For this review, take the finished solid that the model builds, in its own axes (mm). A direction names the side the tool comes from. Give positions to 0.01 mm unless a question says otherwise; leave off trailing zeros. Order: outer loops, then holes, each group sorted by start corner. A loop starts at its lowest first (then second) coordinate and runs counter-clockwise, first axis right, second up. Notation, with made-up numbers: (17, 85.5) - (76, 85.5) arc R30 cw to (76, 117.5) - close; hole circle Ø5 at (48.5, -25.5). An arc over 180 degrees is marked (long way). One line per item, written item: value.
```python
from build123d import *

# Parameters (mm, degrees)
CROQUIS1_R              = 5
SALIENTE_EXTRUIR1_DEPTH = 5
CROQUIS2_R              = 15
SALIENTE_EXTRUIR2_DEPTH = 5
CROQUIS3_R              = 1.5
CORTAR_EXTRUIR1_DEPTH   = 5
REDONDEO1_R             = 1
REDONDEO2_R             = 1


with BuildPart() as part:
    # Croquis1 → Saliente-Extruir1 (new, symmetric)
    with BuildSketch(Plane.XY):
        Circle(CROQUIS1_R)
        with BuildLine():
            Line((-2.236067977, -2), (2.236067977, -2))
            ThreePointArc((2.236067977, -2), (3, 0), (2.236067977, 2))
            Line((2.236067977, 2), (-2.236067977, 2))
            ThreePointArc((-2.236067977, 2), (-3, 0), (-2.236067977, -2))
        make_face(mode=Mode.SUBTRACT)
    extrude(amount=SALIENTE_EXTRUIR1_DEPTH, both=True)

    # Croquis2 → Saliente-Extruir2 (add)
    with BuildSketch(Plane(origin=(0, 0, -5), x_dir=(-1, 0, 0), z_dir=(0, 0, -1))):
        Circle(CROQUIS2_R)
    extrude(amount=SALIENTE_EXTRUIR2_DEPTH)

    # Croquis3 → Cortar-Extruir1 (cut)
    with BuildSketch(Plane.XY.offset(-5)):
        with Locations((-7.5, 7.5)):
            Circle(CROQUIS3_R)
        with Locations((7.5, 7.5)):
            Circle(CROQUIS3_R)
        with Locations((-7.5, -7.5)):
            Circle(CROQUIS3_R)
        with Locations((7.5, -7.5)):
            Circle(CROQUIS3_R)
    extrude(amount=-CORTAR_EXTRUIR1_DEPTH, mode=Mode.SUBTRACT)

    # Redondeo1
    redondeo1_edges = [part.edges().sort_by_distance(p)[0] for p in [
        (15, 0, -5),
    ]]
    fillet(redondeo1_edges, radius=REDONDEO1_R)

    # Redondeo2
    redondeo2_edges = [part.edges().sort_by_distance(p)[0] for p in [
        (-5, 0, 5),
    ]]
    fillet(redondeo2_edges, radius=REDONDEO2_R)


solid = part.part
```
(1) Take a section at B-B (y = 0). Write out the cut boundary in (x, z).
Answers below:
outline: (-15, -10) - (15, -10) - (15, -6) arc R1 ccw to (14, -5) - (5, -5) - (5, 4) arc R1 ccw to (4, 5) - (3, 5) - (3, -5) - (-3, -5) - (-3, 5) - (-4, 5) arc R1 ccw to (-5, 4) - (-5, -5) - (-14, -5) arc R1 ccw to (-15, -6) - close
(2) For P1, Ø5, axis at y = 3.5, z = -1, coming from the +X side; P2, Ø5, axis at x = 7.5, y = -7.5, coming from the +Z side; P3, Ø2, axis at x = 0.5, z = -1, coming from the +Y side, all flat-tipped, find the tip position at first contact; note any pin that passes through.
Answers below:
P1: stops at x = 4.9
P2: stops at z = -5
P3: stops at y = 5
(3) Wall thickness on line 1 (X direction, y = 6.5, z = -9.25); line 2 (Y direction, x = -7.5, z = -7.5); line 3 (Z direction, x = 3.5, y = -8): over which ranges is each line inside the solid? List them lowest first. Write a range as from..to.
Answers below:
line 1: x = -13.52..-8.62, -6.38..6.38, 8.62..13.52
line 2: y = -12.99..-9, -6..6, 9..12.99
line 3: z = -10..-5
(4) Take a section at D-D (x = 7.5). Give the number of separate pieces and of enclosed holes in the cut face, then the cut area to 3 significant figures.
Answers below:
separate pieces: 3
enclosed holes: 0
area: 99.4 mm^2
(5) Draft analysis for pull direction X (two halves, no side actions). For faces 1 (the face through (0, -6, -5)), 2 (the face through (-1.08, -4.88, -0.44)), 3 (the face through (0, 0, -5)), state which applies: pulls with the +X half, pulls with the -X half, needs draft (parallel to the pull), parting line crosses it, or undercut.
Answers below:
face 1: needs draft
face 2: parting line crosses it
face 3: undercut
(6) Take a section at A-A (x = 0). Write out the cut boundary in (y, z), then the cut area to 3 significant figures.
Answers below:
outline: (-15, -10) - (15, -10) - (15, -6) arc R1 ccw to (14, -5) - (5, -5) - (5, 4) arc R1 ccw to (4, 5) - (2, 5) - (2, -5) - (-2, -5) - (-2, 5) - (-4, 5) arc R1 ccw to (-5, 4) - (-5, -5) - (-14, -5) arc R1 ccw to (-15, -6) - close
area: 209 mm^2
(7) Machinability: for faces 4 (the face through (-3, 0, 0)), 5 (the face through (6.3, -8.4, -7.5)), which of the approach directions +Z, -Z, +X, -X, +Y, -Y give a long, thin tool a straight path to every point of the face, cutting with its end or side? Answer none if there is none.
Answers below:
face 4: +Z
face 5: +Z, -Z
(8) Take a section at C-C (z = 2). Write out the cut boundary in (x, y), then the cut area to 3 significant figures.
Answers below:
outline: circle Ø10 at (0, 0); hole (-2.24, -2) - (2.24, -2) arc R3 ccw to (2.24, 2) - (-2.24, 2) arc R3 ccw to start
area: 56.5 mm^2
